Design review of the part built by this model. Coordinates are the model's own, in mm. Coordinates: 2 decimals unless noted, no trailing zeros. Loops run counter-clockwise (first coordinate to the right, second up) from the corner with the lowest first, then second, coordinate; pieces in that order, holes last.
from build123d import *

# Parameters (mm, degrees)
SKETCH3_W           = 150.58
SKETCH3_H           = 100
BOSS_EXTRUDE1_DEPTH = 10
DRAFT1_ANGLE        = 45
SKETCH4_R           = 1.75
CUT_EXTRUDE1_DEPTH  = 15


with BuildPart() as part:
    # Sketch3 → Boss-Extrude1 (new body)
    with BuildSketch(Plane(origin=(0, 0, 0), x_dir=(1, 0, 0), z_dir=(0, 1, 0))):
        with Locations((-1.73528017, -24.11217163)):
            Rectangle(SKETCH3_W, SKETCH3_H)
    extrude(amount=BOSS_EXTRUDE1_DEPTH)

    # Draft1
    draft1_faces = [part.faces().sort_by_distance(p)[0] for p in [
        (73.55471983, 5, 24.11217163),
        (-77.02528017, 5, 24.11217163),
    ]]
    draft(draft1_faces, Plane.ZX.offset(10), DRAFT1_ANGLE)

    # Sketch4 → Cut-Extrude1 (cut)
    with BuildSketch(Plane(origin=(0, 10, 0), x_dir=(1, 0, 0), z_dir=(0, 1, 0))):
        with Locations(Location((69.55471983, 16.88782837, 0), (0, 0, 270))):
            Circle(SKETCH4_R)
        with Locations(Location((-73.02528017, -65.11217163, 0), (0, 0, 270))):
            Circle(SKETCH4_R)
    extrude(amount=-CUT_EXTRUDE1_DEPTH, mode=Mode.SUBTRACT)


solid = part.part
Q1. The part is to be moulded in two halves that separate along X. For faces 1 (the flat face through (-3, 0, 23)), 2 (the flat face through (-82.095, 4.93, 24.812)), 3 (the cylindrical face through (67.846, 5.07, -17.267)), say which applies: pulls with the +X half, pulls with the -X half, needs draft (parallel to the pull), parting line crosses it, or undercut.
Q2. Take a section at A-A, the plane y = 8.5. Write out the cut boundary in (x, z).
Q3. Clearance check with flat-ended pins moving along their axes: pin 1 Ø1 at (y, z) = (9, 46) entering from +X; pin 2 Ø1 at (y, z) = (4.5, 19.5) entering from -X; pin 3 Ø1.5 at (y, z) = (9, 57) entering from +X. State where each tip first meets the part, or that it passes through.
Q4. For line 1 (X direction, y = 5.25, z = 24.5); line 2 (X direction, y = 2, z = -15), list the stretches that pass through material, from the lowest coordinate up.
Q5. Take a section at B-B, the plane z = 33. Write out the cut boundary in (x, y), then the cut area to 3 significant figures.
Entries:
1. face 1: needs draft
1. face 2: pulls with the -X half
1. face 3: undercut
2. outline: (-78.53, -25.89) - (75.05, -25.89) - (75.05, 74.11) - (-78.53, 74.11) - close; hole circle Ø3.5 at (-73.03, 65.11); hole circle Ø3.5 at (69.55, -16.89)
3. pin 1: stops at x = 75.05
3. pin 2: stops at x = -83.03
3. pin 3: stops at x = 75.3
4. line 1: x = -81.78 to 78.3
4. line 2: x = -85.03 to 81.55
5. outline: (-87.03, 0) - (83.55, 0) - (73.55, 10) - (-77.03, 10) - close
5. area: 1,610 mm2
